from build123d import *

# Parameters (mm, degrees)
SZKIC1_R                    = 7.5
SZKIC1_R_2                  = 4
DODANIE_WYCI_GNI_CIE1_DEPTH = 12
SZKIC2_R                    = 6.75
WYTNIJ_WYCI_GNI_CIE1_DEPTH  = 1.25
SZKIC3_R                    = 4.5
SZKIC3_R_2                  = 4
DODANIE_WYCI_GNI_CIE2_DEPTH = 0.5
SFAZOWANIE1_SIZE            = 0.35
SFAZOWANIE1_SIZE2           = 0.606217783
SZKIC4_R                    = 7.5
SZKIC4_R_2                  = 7.125
WYTNIJ_WYCI_GNI_CIE2_DEPTH  = 1.25
SFAZOWANIE2_SIZE            = 0.35
SFAZOWANIE2_SIZE2           = 0.606217783


with BuildPart() as part:
    # Szkic1 → Dodanie-wyciągnięcie1 (new, symmetric)
    with BuildSketch(Plane.XY):
        Circle(SZKIC1_R)
        Circle(SZKIC1_R_2, mode=Mode.SUBTRACT)
    extrude(amount=DODANIE_WYCI_GNI_CIE1_DEPTH, both=True)

    # Szkic2 → Wytnij-wyciągnięcie1 (cut)
    with BuildSketch(Plane.XY.offset(12)):
        Circle(SZKIC2_R)
    wytnij_wyci_gni_cie1 = extrude(amount=-WYTNIJ_WYCI_GNI_CIE1_DEPTH, mode=Mode.SUBTRACT)

    # Szkic3 → Dodanie-wyciągnięcie2 (add)
    with BuildSketch(Plane.XY.offset(10.75)):
        Circle(SZKIC3_R)
        Circle(SZKIC3_R_2, mode=Mode.SUBTRACT)
    dodanie_wyci_gni_cie2 = extrude(amount=DODANIE_WYCI_GNI_CIE2_DEPTH)

    # Sfazowanie1
    sfazowanie1_edges = [part.edges().sort_by_distance(p)[0] for p in [
        (-6.75, 0, 12),
    ]]
    sfazowanie1_side = [part.faces().sort_by_distance(p)[0] for p in [
        (-7.287867966, 0, 12),
    ]]
    chamfer(sfazowanie1_edges, length=SFAZOWANIE1_SIZE, length2=SFAZOWANIE1_SIZE2, reference=sfazowanie1_side[0])

    # Szkic4 → Wytnij-wyciągnięcie2 (cut)
    with BuildSketch(Plane.XY.offset(8)):
        Circle(SZKIC4_R)
        Circle(SZKIC4_R_2, mode=Mode.SUBTRACT)
    wytnij_wyci_gni_cie2 = extrude(amount=-WYTNIJ_WYCI_GNI_CIE2_DEPTH, mode=Mode.SUBTRACT)

    # Lustro4: Wytnij-wyciągnięcie1, Dodanie-wyciągnięcie2, Wytnij-wyciągnięcie2 across plane
    add(wytnij_wyci_gni_cie1.mirror(Plane.XY), mode=Mode.SUBTRACT)
    add(dodanie_wyci_gni_cie2.mirror(Plane.XY))
    add(wytnij_wyci_gni_cie2.mirror(Plane.XY), mode=Mode.SUBTRACT)

    # Sfazowanie2
    sfazowanie2_edges = [part.edges().sort_by_distance(p)[0] for p in [
        (-6.75, 0, -12),
    ]]
    sfazowanie2_side = [part.faces().sort_by_distance(p)[0] for p in [
        (-7.287867966, 0, -12),
    ]]
    chamfer(sfazowanie2_edges, length=SFAZOWANIE2_SIZE, length2=SFAZOWANIE2_SIZE2, reference=sfazowanie2_side[0])


solid = part.part
CAD build for the part. Positions are in the model's coordinates, mm. A direction names the side the tool comes from. Round coordinates to 2 decimals unless told otherwise and drop trailing zeros. Loops run counter-clockwise (first coordinate to the right, second up) from the corner with the lowest first, then second, coordinate; pieces in that order, holes last.
(1) Two-plate mould, pull along Z, no slides. Class faces 1 (the cylindrical face through (6.58, -2.73, -7.38)), 2 (the flat face through (4.4, 1.6, 10.75)), 3 (the cylindrical face through (-1.46, -6.59, -11.08)): +Z half, -Z half, draft (parallel to the pull), parting line (faces both ways), or undercut.
(2) Drop flat-ended pins along their axis: pin 1 (7 mm diameter, centred on x = -3, y = 1.5, fed in from -Z); pin 2 (5 mm diameter, centred on x = -1, y = -3.5, fed in from +Z); pin 3 (5 mm diameter, centred on y = 3, z = 1, fed in from +X); pin 4 (5 mm diameter, centred on x = 1, y = 6, fed in from +Z). Give the stop position or say it passes through.
(3) Wall check: line 1 along Y through (x, z) = (0, -10.9); line 2 along Z through (x, y) = (-5.5, 5); line 3 along Y through (x, z) = (0, 2.5). Give the ranges that are in metal, low to high.
(4) Cut at A-A (z = -1.5). Give the cut face in (x, y), plus the area to 3 significant figures.
(5) Which spindle directions (+Z, -Z, +X, -X, +Y, -Y) get a long thin tool onto all of the face, cutting with end or side? Do faces 4 (the cylindrical face through (6.58, -2.73, 7.38)), 5 (the cylindrical face through (-0.59, 4.46, 11)), 6 (the cylindrical face through (-7.493, 0.33, 10.028)), 7 (the flat face through (-3, -3, -11.25)). Say none if no direction does.
Findings below:
1. face 1: undercut
1. face 2: +Z half
1. face 3: draft
2. pin 1: stops at z = -11.57
2. pin 2: stops at z = 11.25
2. pin 3: stops at x = 7.48
2. pin 4: stops at z = 12
3. line 1: y = -7.5 to -6.75, -4.5 to -4, 4 to 4.5, 6.75 to 7.5
3. line 2: z = -12 to -8, -6.75 to 6.75, 8 to 12
3. line 3: y = -7.5 to -4, 4 to 7.5
4. outline: circle Ø15 at (0, 0); hole circle Ø8 at (0, 0)
4. area: 126 mm2
5. face 4: none
5. face 5: +Z
5. face 6: +Z, -Z
5. face 7: -Z
